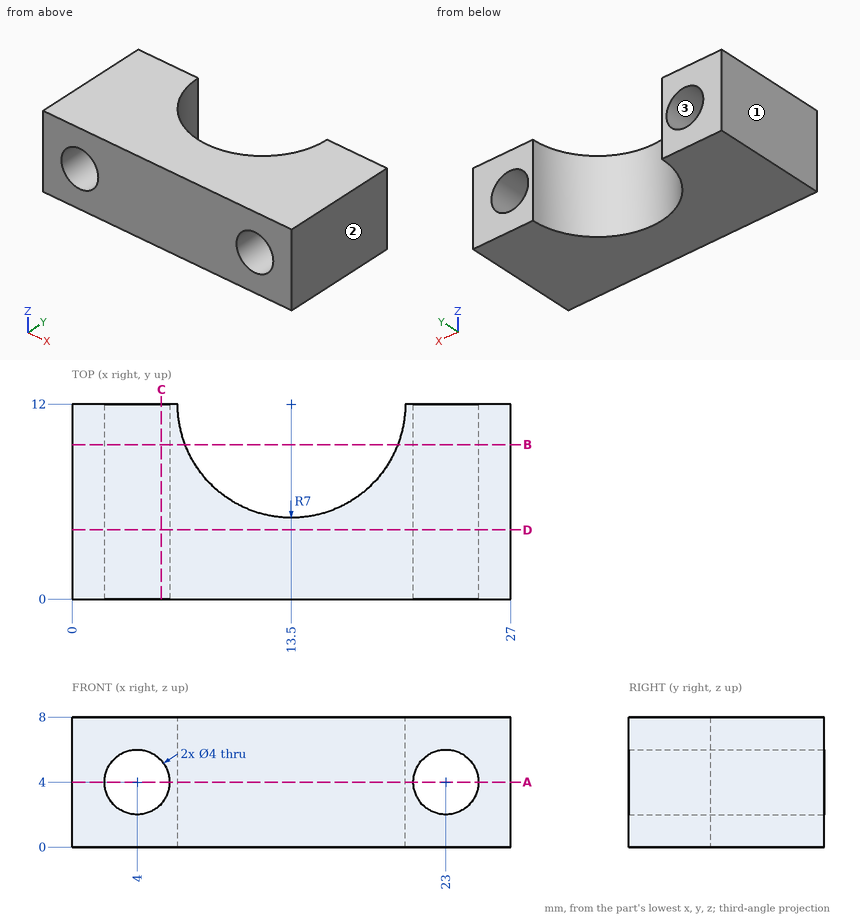
Source: three-view drawing plus pictorial views. Frame: mm from the lowest corner of the part. Round coordinates to 2 decimals unless told otherwise and drop trailing zeros. Loops run counter-clockwise (first coordinate to the right, second up) from the corner with the lowest first, then second, coordinate; pieces in that order, holes last. Notation, with made-up numbers: M 72.25,-19.5 L 121.25,-19.5 A23 ccw 121.25,-4.5 Z; hole C 75.25,20 d6. An arc over 180 degrees is marked long. Answer as CSV lines item,"result". Start each with the question number.
(1) First-contact query: pin 1 (1.5 mm diameter, centred on x = 13, z = 3, fed in from +Y); pin 2 (1 mm diameter, centred on x = 10, y = 7, fed in from -Z). Flat tips, straight axial feed; report the tip coordinate or a pass-through.
(2) Section A-A, the plane z = 4. Output: boundary loops of the cut face in (x, y), plus the area to 3 significant figures.
(3) Draft query along X for the marked faces 1, 2 and 3. Return one class per face: released by +X, released by -X, zero draft, split by the parting line, or undercut.
(4) Line query: line 1 (X direction, y = 3.5, z = 4); line 2 (X direction, y = 10.75, z = 4.75); line 3 (X direction, y = 9.75, z = 5.5). Output: solid intervals per line, ascending. Write a range as [from, to].
(5) Section D-D, the plane y = 4.25. Output: boundary loops of the cut face in (x, z), plus the area to 3 significant figures.
(6) Section B-B, the plane y = 9.5. Output: boundary loops of the cut face in (x, z), plus the area to 3 significant figures.
(7) Section C-C, the plane x = 5.5. Output: boundary loops of the cut face in (y, z).
Values found:
1,pin 1,"stops at y = 5.11"
1,pin 2,"passes through"
2,outline,"M 0,0 L 2,0 L 2,12 L 0,12 Z; M 6,0 L 21,0 L 21,12 L 20.5,12 A7 cw 6.5,12 L 6,12 Z; M 25,0 L 27,0 L 27,12 L 25,12 Z"
2,area,"151 mm²"
3,face 1,"released by -X"
3,face 2,"released by +X"
3,face 3,"undercut"
4,line 1,"x = [0, 2], [6, 21], [25, 27]"
4,line 2,"x = [0, 2.15], [5.85, 6.61], [20.39, 21.15], [24.85, 27]"
4,line 3,"x = [0, 2.68], [5.32, 6.87], [20.13, 21.68], [24.32, 27]"
5,outline,"M 0,0 L 27,0 L 27,8 L 0,8 Z; hole C 4,4 d4; hole C 23,4 d4"
5,area,"191 mm²"
6,outline,"M 0,0 L 6.96,0 L 6.96,8 L 0,8 Z; M 20.04,0 L 27,0 L 27,8 L 20.04,8 Z; hole C 4,4 d4; hole C 23,4 d4"
6,area,"86.3 mm²"
7,outline,"M 0,0 L 12,0 L 12,2.68 L 0,2.68 Z; M 0,5.32 L 12,5.32 L 12,8 L 0,8 Z"
